For this review, take the finished solid that the model builds, in its own axes (mm). Give positions to 0.01 mm unless a question says otherwise; leave off trailing zeros. Order: outer loops, then holes, each group sorted by start corner. A loop starts at its lowest first (then second) coordinate and runs counter-clockwise, first axis right, second up. Notation, with made-up numbers: (24.5, 16) - (60.5, 16) arc R13 cw to (60.5, 27) - close; hole circle Ø10 at (-9, -33). An arc over 180 degrees is marked (long way). Put each result on its own line as item: value. Start each with the question number.
```python
from build123d import *

# Parameters (mm, degrees)
SKETCH1_W           = 647.7
SKETCH1_H           = 85.344
BOSS_EXTRUDE1_DEPTH = 3.175
SKETCH2_W           = 43.18
SKETCH2_H           = 2.54
BOSS_EXTRUDE2_DEPTH = 3.175
SKETCH3_W           = 137.668
SKETCH3_H           = 16.764
BOSS_EXTRUDE3_DEPTH = 3.175


with BuildPart() as part:
    # Sketch1 → Boss-Extrude1 (new body)
    with BuildSketch(Plane.XY):
        with Locations((323.85, 42.672)):
            Rectangle(SKETCH1_W, SKETCH1_H)
    extrude(amount=-BOSS_EXTRUDE1_DEPTH)

    # Sketch2 → Boss-Extrude2 (add)
    with BuildSketch(Plane.XY):
        with Locations((626.11, -1.27)):
            Rectangle(SKETCH2_W, SKETCH2_H)
    extrude(amount=-BOSS_EXTRUDE2_DEPTH)

    # Sketch3 → Boss-Extrude3 (add)
    with BuildSketch(Plane.XY):
        with Locations((118.3894, 93.726)):
            Rectangle(SKETCH3_W, SKETCH3_H)
    extrude(amount=-BOSS_EXTRUDE3_DEPTH)


solid = part.part
```
1. Clearance check with a flat-ended pin moving along its axis: pin 1 (1.6 mm diameter, centred on x = 35, z = -1.5, fed in from +Y). State where the tip first meets the part, or that it passes through.
2. Add section B-B, the plane x = 157.5. Give the boundary of the cut face in (y, z) (3 decimals), then the cut area to 3 significant figures.
3. Add section A-A, the plane z = -0.95. Give the boundary of the cut face in (x, y).
4. Add section C-C, the plane y = 91. Give the boundary of the cut face in (x, z) (3 decimals).
5. Wall thickness on line 1 (Y direction, x = 227.5, z = -2.6); line 2 (Y direction, x = 114, z = -0.65); line 3 (X direction, y = 86, z = -3): over which ranges is each line inside the solid? List them lowest first. Write a range as from..to.
Found:
1. pin 1: stops at y = 85.34
2. outline: (0, -3.175) - (102.108, -3.175) - (102.108, 0) - (0, 0) - close
2. area: 324 mm^2
3. outline: (0, 0) - (604.52, 0) - (604.52, -2.54) - (647.7, -2.54) - (647.7, 85.34) - (187.22, 85.34) - (187.22, 102.11) - (49.56, 102.11) - (49.56, 85.34) - (0, 85.34) - close
4. outline: (49.555, -3.175) - (187.223, -3.175) - (187.223, 0) - (49.555, 0) - close
5. line 1: y = 0..85.34
5. line 2: y = 0..102.11
5. line 3: x = 49.56..187.22
